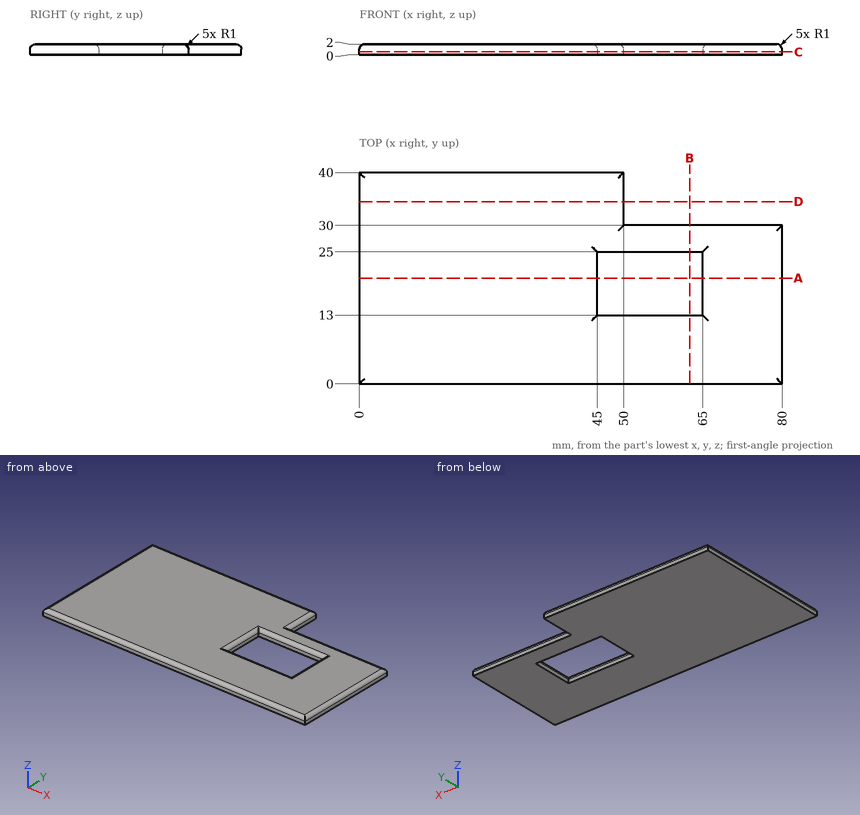
Check sheet for the drawn part. Datum: minimum x, y, z corner. Units: mm. Give positions to 0.01 mm unless a question says otherwise; leave off trailing zeros. Write each loop counter-clockwise with the first axis right and the second up, starting at its lowest first coordinate (ties: lowest second). Pieces come first, ordered by that corner, then holes. Notation, with made-up numbers: (32.5, 23.5) - (40.5, 23.5) arc R20 ccw to (40.5, 32.5) - close; hole circle Ø8 at (55, 17.5). An arc over 180 degrees is marked (long way). Put each result on its own line as item: value.
1. Thickness scan on line 1 (X direction, y = 21, z = 0.45); line 2 (Y direction, x = 46.5, z = 0.6); line 3 (Y direction, x = 20.5, z = 1.1). Record the ranges inside material, lowest first.
Ans:
line 1: x = 0 to 45, 65 to 80
line 2: y = 0 to 13, 25 to 40
line 3: y = 0.01 to 39.99
2. Go/stop test with flat-tipped pins: pin 1 (1.1 mm diameter, centred on y = 34.5, z = 0.5, fed in from +X); pin 2 (8 mm diameter, centred on x = 20.5, y = 6, fed in from -Z); pin 3 (1.1 mm diameter, centred on x = 53.5, z = 0.5, fed in from +Y). Record where each tip stops, or that it passes through.
Ans:
pin 1: stops at x = 50
pin 2: stops at z = 0
pin 3: stops at y = 30
3. Sectioned sample at D-D, the plane y = 34.5. Enter the section's corners in (x, z).
Ans:
outline: (0, 0) - (50, 0) - (50, 1) arc R1 ccw to (49, 2) - (1, 2) arc R1 ccw to (0, 1) - close
4. Sectioned sample at B-B, the plane x = 62.5. Enter the section's corners in (y, z).
Ans:
outline: (0, 0) - (13, 0) - (13, 1) arc R1 ccw to (12, 2) - (1, 2) arc R1 ccw to (0, 1) - close; (25, 0) - (30, 0) - (30, 1) arc R1 ccw to (29, 2) - (26, 2) arc R1 ccw to (25, 1) - close
5. Sectioned sample at C-C, the plane z = 0.5. Enter the section's corners in (x, y), plus the area to 3 significant figures.
Ans:
outline: (0, 0) - (80, 0) - (80, 30) - (50, 30) - (50, 40) - (0, 40) - close; hole (45, 13) - (65, 13) - (65, 25) - (45, 25) - close
area: 2,660 mm²
6. Sectioned sample at A-A, the plane y = 20. Enter the section's corners in (x, z).
Ans:
outline: (0, 0) - (45, 0) - (45, 1) arc R1 ccw to (44, 2) - (1, 2) arc R1 ccw to (0, 1) - close; (65, 0) - (80, 0) - (80, 1) arc R1 ccw to (79, 2) - (66, 2) arc R1 ccw to (65, 1) - close
